```python
from build123d import *

# Parameters (mm, degrees)
EXTRUDE_X1_DEPTH          = 25
CUT_EXTRUDE_X2_DEPTH      = 337.68365599
CUT_EXTRUDE_X2_DEPTH_BACK = 337.68365599
SHELL_S1_T                = -5
SKETCH_C_R                = 22.5
EXTRUDE_X3_DEPTH          = 35
SKETCH_D_R                = 17.5
CUT_EXTRUDE_X5_DEPTH      = 1
CUT_EXTRUDE_START         = -1
SKETCH_E_R                = 17.5
CUT_EXTRUDE_X6_DEPTH      = 1
CUT_EXTRUDE_X7_DEPTH      = 338.471850678
FILLET_F1_R               = 4


with BuildPart() as part:
    # Sketch A → Extrude X1 (new body)
    with BuildSketch(Plane(origin=(0, 0, 0), x_dir=(1, 0, 0), z_dir=(0, 1, 0))):
        Polygon((0.604805244, 22.491869878), (335, 13.5), (335, -13.5), (0.604805244, -22.491869878), align=None)
    extrude(amount=EXTRUDE_X1_DEPTH)

    # Sketch B → Cut-Extrude X2 (cut, two sides: drawn at the far end of the back side and taken through both)
    with BuildSketch(Plane.XY.offset(-CUT_EXTRUDE_X2_DEPTH_BACK)):
        Polygon((335, 12.5), (140, 0), (140, -74.146668182), (362.466184873, -74.146668182), (356.911911272, 12.5), align=None)
    extrude(amount=CUT_EXTRUDE_X2_DEPTH + CUT_EXTRUDE_X2_DEPTH_BACK, mode=Mode.SUBTRACT)

    # Shell S1
    shell_s1_openings = [part.faces().sort_by_distance(p)[0] for p in [
        (153.878711478, 25, 0),
        (0.604805244, 12.5, 0),
    ]]
    offset(amount=SHELL_S1_T, openings=shell_s1_openings, kind=Kind.INTERSECTION)

    # Sketch C → Extrude X3 (add)
    with BuildSketch(Plane(origin=(0, 0, 0), x_dir=(1, 0, 0), z_dir=(0, 1, 0))):
        with Locations(Location((0, 0, 0), (0, 0, 88.459690565))):
            Circle(SKETCH_C_R)
    extrude(amount=EXTRUDE_X3_DEPTH)

    # Sketch D → Cut-Extrude X5 (cut)
    with BuildSketch(Plane(origin=(0, 35, 0), x_dir=(1, 0, 0), z_dir=(0, 1, 0))):
        with Locations(Location((0, 0, 0), (0, 0, 270))):
            Circle(SKETCH_D_R)
    extrude(amount=-CUT_EXTRUDE_X5_DEPTH, mode=Mode.SUBTRACT)

    # Sketch E → Cut-Extrude X6 (cut)
    with BuildSketch(Plane.XZ.offset(CUT_EXTRUDE_START)):
        with Locations(Location((0, 0, 0), (0, 0, 90))):
            Circle(SKETCH_E_R)
    extrude(amount=CUT_EXTRUDE_X6_DEPTH, mode=Mode.SUBTRACT)

    # Sketch F → Cut-Extrude X7 (cut, through all)
    with BuildSketch(Plane(origin=(0, 1, 0), x_dir=(1, 0, 0), z_dir=(0, 1, 0))):
        Polygon((0, 15.556349186), (-15.556349186, 0), (0, -15.556349186), (15.556349186, 0), align=None)
    extrude(amount=CUT_EXTRUDE_X7_DEPTH, mode=Mode.SUBTRACT)

    # Fillet F1
    fillet_f1_edges = [part.edges().sort_by_distance(p)[0] for p in [
        (330, 21.094874747, 8.6326424),
        (330, 21.094874747, -8.6326424),
        (14.607429601, 15, -17.11353267),
        (14.607429601, 15, 17.11353267),
    ]]
    fillet(fillet_f1_edges, radius=FILLET_F1_R)


solid = part.part
```
Geometry: final body of the model. Coordinates: model frame, mm. A direction names the side the tool comes from. Give positions to 0.01 mm unless a question says otherwise; leave off trailing zeros. Loops run counter-clockwise (first coordinate to the right, second up) from the corner with the lowest first, then second, coordinate; pieces in that order, holes last. Notation, with made-up numbers: (32.25, 47.5) - (90.25, 47.5) arc R17 cw to (90.25, 72.5) - close; hole circle Ø3 at (28, 7.25). An arc over 180 degrees is marked (long way). Answer as CSV lines item,"result". Start each with the question number.
(1) Reachability of faces 1 (the face through (19.71, 14.86, -14.91)), 2 (the face through (14, 35, -11)), 3 (the face through (7.887, 17.269, -7.669)) from +Z, -Z, +X, -X, +Y, -Y: full face, straight path, thin tool, end or side. Return the list, or none.
(2) Section query C-C (x = 268). Output: boundary loops of the cut face in (y, z), and give its area (3 significant figures).
(3) Ray query, line 1 along X through (y, z) = (34.5, 0); line 2 along Y through (x, z) = (78, 8); line 3 along Z through (x, y) = (315.5, 24). Return the intervals inside material, ascending. Write a range as [from, to].
(4) Pin query (flat end, axial travel): P1, Ø17, axis at x = 77.5, z = -6.5, coming from the +Y side; P2, Ø10, axis at x = 192.5, y = 27.5, coming from the +Z side; P3, Ø6, axis at x = 236.5, y = 20, coming from the -Z side. Return the tip coordinate at first contact, or that it passes through.
(5) Mould query, pull axis Z, two halves, no side actions, for faces 4 (the face through (10.648, 0.507, -13.887)), 5 (the face through (335, 19, 0)). Classes: +Z half, -Z half, draft (parallel to the pull), parting line (faces both ways), or undercut.
(6) Section query A-A (y = 29). Output: boundary loops of the cut face in (x, z).
(7) Section query B-B (x = 52). Output: boundary loops of the cut face in (y, z).
Worked answers:
1,face 1,"+Y"
1,face 2,"+Z, -Z, +X, -X, +Y"
1,face 3,"+Y, -Y"
2,outline,"(8.21, -15.3) - (25, -15.3) - (25, -10.3) - (13.22, -10.3) - (13.22, 10.3) - (25, 10.3) - (25, 15.3) - (8.21, 15.3) - close"
2,area,"271 mm^2"
3,line 1,"x = [-22.5, -17.5], [17.5, 22.5]"
3,line 2,"y = [0, 5]"
3,line 3,"z = [-14.02, -9.02], [9.02, 14.02]"
4,P1,"stops at y = 5"
4,P2,"stops at z = 17.45"
4,P3,"stops at z = -16.23"
5,face 4,"undercut"
5,face 5,"draft"
6,outline,"circle Ø45 at (0, 0); hole (-15.56, 0) - (0, -15.56) - (15.56, 0) - (0, 15.56) - close"
7,outline,"(0, -21.11) - (25, -21.11) - (25, -16.11) - (5, -16.11) - (5, 16.11) - (25, 16.11) - (25, 21.11) - (0, 21.11) - close"
